The listing builds one solid part. Answer for the finished solid, in the listing's coordinates (mm). Give positions to 0.01 mm unless a question says otherwise; leave off trailing zeros. Loops run counter-clockwise (first coordinate to the right, second up) from the corner with the lowest first, then second, coordinate; pieces in that order, holes last. Notation, with made-up numbers: (-24.75, 76) - (10.25, 76) arc R23 cw to (10.25, 113) - close; hole circle Ø7 at (37.25, -25.5). An arc over 180 degrees is marked (long way). Write item = value, one per line. Start each with the question number.
1) Consider probe 1 along Y at (x, z) = (1.8, 0.2); probe 2 along X at (y, z) = (5, 0.05). Determine where each line is inside the solid, lowest interval first.
2) The part is cut by section B-B on x = -0.3. Write down the section's boundary in (y, z).
3) The part is cut by section A-A on y = 0. Write down the section's boundary in (x, z).
4) The part is cut by section D-D on y = 2.5. Write down the section's boundary in (x, z), plus the area to 3 significant figures.
5) The part is cut by section C-C on z = 0.15. Write down the section's boundary in (x, y).
from build123d import *

# Parameters (mm, degrees)
BOSS_EXTRUDE1_DEPTH = 0.1
SKETCH3_R           = 2.1
BOSS_EXTRUDE2_DEPTH = 0.32
SKETCH4_R           = 2
CUT_EXTRUDE1_DEPTH  = 1.32
SKETCH5_W           = 0.2
SKETCH5_H           = 0.897152977
CUT_EXTRUDE2_DEPTH  = 1.32


with BuildPart() as part:
    # Sketch1 → Boss-Extrude1 (new body)
    with BuildSketch(Plane.XY):
        with BuildLine():
            Line((0, 6.75), (0.1, 6.75))
            Line((0.1, 6.75), (0.5, 2.347338919))
            ThreePointArc((0.5, 2.347338919), (0, -2.4), (-0.5, 2.347338919))
            Line((-0.5, 2.347338919), (-0.1, 6.75))
            Line((-0.1, 6.75), (0, 6.75))
        make_face()
    extrude(amount=BOSS_EXTRUDE1_DEPTH)

    # Sketch3 → Boss-Extrude2 (add)
    with BuildSketch(Plane.XY):
        Circle(SKETCH3_R)
    extrude(amount=BOSS_EXTRUDE2_DEPTH)

    # Sketch4 → Cut-Extrude1 (cut, through all)
    with BuildSketch(Plane.XY):
        Circle(SKETCH4_R)
    extrude(amount=CUT_EXTRUDE1_DEPTH, mode=Mode.SUBTRACT)

    # Sketch5 → Cut-Extrude2 (cut, through all)
    with BuildSketch(Plane.XY):
        with Locations((0, -2.259612308)):
            Rectangle(SKETCH5_W, SKETCH5_H)
    extrude(amount=CUT_EXTRUDE2_DEPTH, mode=Mode.SUBTRACT)


solid = part.part
Answer below:
q1.probe_1 = -1.08 to -0.87, 0.87 to 1.08
q1.probe_2 = -0.26 to 0.26
q2.outline = (-2.38, 0) - (-1.98, 0) - (-1.98, 0.32) - (-2.08, 0.32) - (-2.08, 0.1) - (-2.38, 0.1) - close; (1.98, 0) - (4.55, 0) - (4.55, 0.1) - (2.08, 0.1) - (2.08, 0.32) - (1.98, 0.32) - close
q3.outline = (-2.4, 0) - (-2, 0) - (-2, 0.32) - (-2.1, 0.32) - (-2.1, 0.1) - (-2.4, 0.1) - close; (2, 0) - (2.4, 0) - (2.4, 0.1) - (2.1, 0.1) - (2.1, 0.32) - (2, 0.32) - close
q4.outline = (-0.49, 0) - (0.49, 0) - (0.49, 0.1) - (-0.49, 0.1) - close
q4.area = 0.0972 mm2
q5.outline = (-0.1, -2.1) - (-0.1, -2) arc R2 cw (long way) to (0.1, -2) - (0.1, -2.1) arc R2.1 ccw (long way) to start
